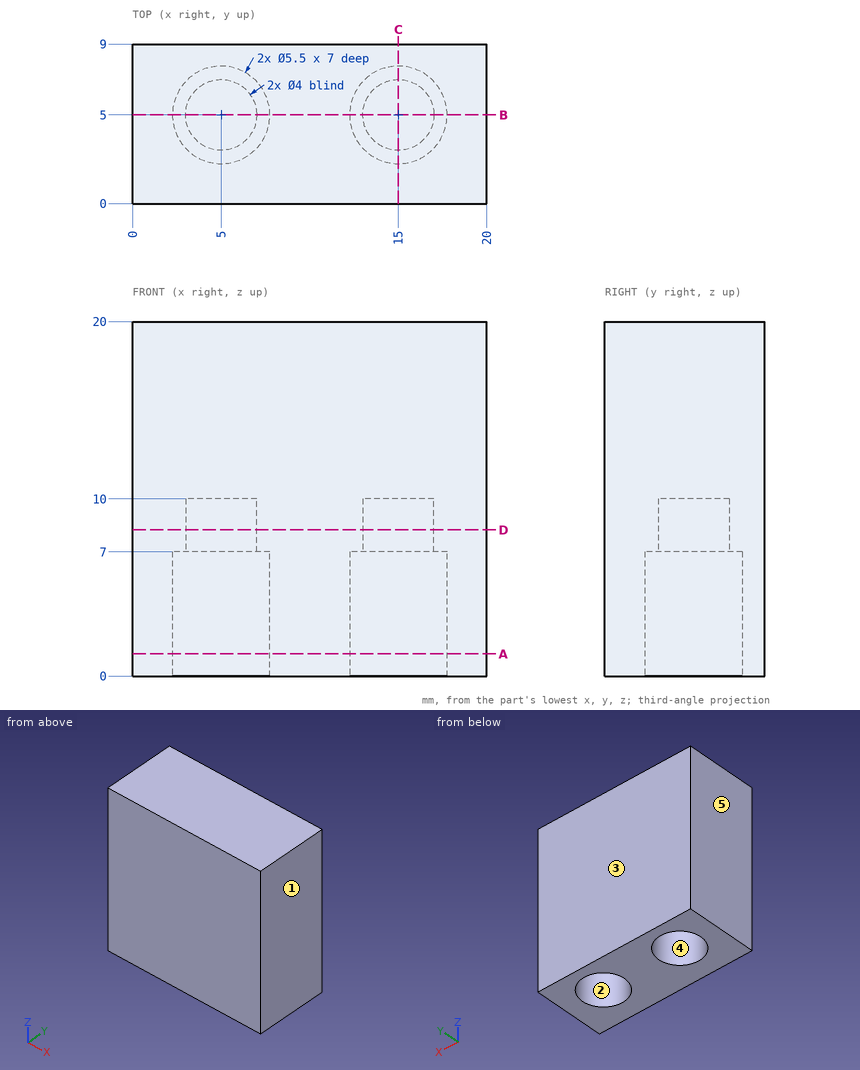
Can you work these out from the drawing? Everything is in mm from the part's minimum corner. A direction names the side the tool comes from. Give positions to 0.01 mm unless a question says otherwise; leave off trailing zeros. Order: outer loops, then holes, each group sorted by start corner. A loop starts at its lowest first (then second) coordinate and runs counter-clockwise, first axis right, second up.
Item 1: I need wall thicknesses on line 1 (X direction, y = 5, z = 8.05); line 2 (Y direction, x = 15, z = 2); line 3 (X direction, y = 4.5, z = 6). Which ranges of each line are inside material? Lowest first, please.
Item 2: If we section it at C-C, the plane x = 15: Write out the boundary of the cut face in (y, z).
Item 3: If we section it at A-A, the plane z = 1.25: Write out the boundary of the cut face in (x, y), plus the area to 3 significant figures.
Item 4: If we section it at D-D, the plane z = 8.25: Write out the boundary of the cut face in (x, y).
Item 5: If we mould it in two halves opening along X, with no side actions, what happens to the marked faces 1, 2 and 3? For each: pulls with the +X half, pulls with the -X half, needs draft (parallel to the pull), parting line crosses it, or undercut.
Item 6: For the marked faces 4 and 5, which set-ups out of +Z, -Z, +X, -X, +Y, -Y let a thin tool reach every point of the face, with its end or its side?
Item 7: If we section it at B-B, the plane y = 5: Write out the boundary of the cut face in (x, z).
Item 8: I'm going to push a flat-ended pin straight in: pin 1 (3 mm diameter, centred on x = 15, y = 5, fed in from -Z). Where does the tip first touch, or does it pass through?
Values:
1. line 1: x = 0 to 3, 7 to 13, 17 to 20
1. line 2: y = 0 to 2.25, 7.75 to 9
1. line 3: x = 0 to 2.3, 7.7 to 12.3, 17.7 to 20
2. outline: (0, 0) - (2.25, 0) - (2.25, 7) - (3, 7) - (3, 10) - (7, 10) - (7, 7) - (7.75, 7) - (7.75, 0) - (9, 0) - (9, 20) - (0, 20) - close
3. outline: (0, 0) - (20, 0) - (20, 9) - (0, 9) - close; hole circle Ø5.5 at (5, 5); hole circle Ø5.5 at (15, 5)
3. area: 132 mm2
4. outline: (0, 0) - (20, 0) - (20, 9) - (0, 9) - close; hole circle Ø4 at (5, 5); hole circle Ø4 at (15, 5)
5. face 1: pulls with the +X half
5. face 2: undercut
5. face 3: needs draft
6. face 4: -Z
6. face 5: +Z, -Z, -X, +Y, -Y
7. outline: (0, 0) - (2.25, 0) - (2.25, 7) - (3, 7) - (3, 10) - (7, 10) - (7, 7) - (7.75, 7) - (7.75, 0) - (12.25, 0) - (12.25, 7) - (13, 7) - (13, 10) - (17, 10) - (17, 7) - (17.75, 7) - (17.75, 0) - (20, 0) - (20, 20) - (0, 20) - close
8. pin 1: stops at z = 10
